The listing builds one solid part. Answer for the finished solid, in the listing's coordinates (mm). Face numbers are marked on the shaded views. A direction names the side the tool comes from. Coordinates: 2 decimals unless noted, no trailing zeros. Order: outer loops, then holes, each group sorted by start corner. A loop starts at its lowest first (then second) coordinate and runs counter-clockwise, first axis right, second up. Notation, with made-up numbers: (58, 19.5) -> (91, 19.5) arc R34 cw to (91, 50.5) -> close; hole circle Ø11 at (-16.75, 63.25). An arc over 180 degrees is marked (long way). Answer in a Markdown table with one row per item.
```python
from build123d import *

# Parameters (mm, degrees)
SKETCH1_W                       = 16
SKETCH1_H                       = 8
BOSS_EXTRUDE1_DEPTH             = 3
SHELL1_T                        = -1
BOSS_EXTRUDE2_DEPTH             = 11
CUT_EXTRUDE1_DEPTH              = 13
SKETCH4_R                       = 1.2
BOSS_EXTRUDE3_DEPTH             = 3
BOSS_EXTRUDE3_DIRECTION_2_REACH = 8.299


with BuildPart() as part:
    # Sketch1 → Boss-Extrude1 (new body)
    with BuildSketch(Plane(origin=(0, 0, 0), x_dir=(1, 0, 0), z_dir=(0, 1, 0))):
        Rectangle(SKETCH1_W, SKETCH1_H)
    extrude(amount=BOSS_EXTRUDE1_DEPTH)

    # Shell1
    shell1_openings = [part.faces().sort_by_distance(p)[0] for p in [
        (0, 0, 0),
    ]]
    offset(amount=SHELL1_T, openings=shell1_openings, kind=Kind.INTERSECTION)

    # Sketch2 → Boss-Extrude2 (add)
    with BuildSketch(Plane(origin=(0, 3, 0), x_dir=(1, 0, 0), z_dir=(0, 1, 0))):
        with BuildLine():
            Line((-4, 4), (4, 4))
            Line((4, 4), (4, 2.5))
            Line((4, 2.5), (2, 2.5))
            ThreePointArc((2, 2.5), (0, 1.5), (-2, 2.5))
            Line((-2, 2.5), (-4, 2.5))
            Line((-4, 2.5), (-4, 4))
        make_face()
    extrude(amount=BOSS_EXTRUDE2_DEPTH)

    # Sketch3 → Cut-Extrude1 (cut, through all)
    with BuildSketch(Plane(origin=(4, 0, 0), x_dir=(0, 0, -1), z_dir=(1, 0, 0))):
        Polygon((1.5, 14), (1.5, 10), (3.25, 14), align=None)
    extrude(amount=-CUT_EXTRUDE1_DEPTH, mode=Mode.SUBTRACT)

    # Sketch4 → Boss-Extrude3 (add)
    with BuildSketch(Plane(origin=(0, 1.055737705, 2.413114754), x_dir=(1, 0, 0), z_dir=(0, 0.400818834, 0.916157335))):
        with Locations((0, 13.193478025)):
            Circle(SKETCH4_R)
    extrude(amount=BOSS_EXTRUDE3_DEPTH)

    # Sketch4 → Boss-Extrude3 direction 2 (add, up to next)
    with BuildSketch(Plane(origin=(0, 1.055737705, 2.413114754), x_dir=(1, 0, 0), z_dir=(0, 0.400818834, 0.916157335)), mode=Mode.PRIVATE) as boss_extrude3_direction_2_sk1:
        with Locations((0, 13.193478025)):
            Circle(SKETCH4_R)
    boss_extrude3_direction_2_tool1 = extrude(boss_extrude3_direction_2_sk1.sketch, amount=-BOSS_EXTRUDE3_DIRECTION_2_REACH, mode=Mode.PRIVATE) - part.part
    add(boss_extrude3_direction_2_tool1.solids().sort_by_distance((0, 13.143039, -2.87508))[0])


solid = part.part
```
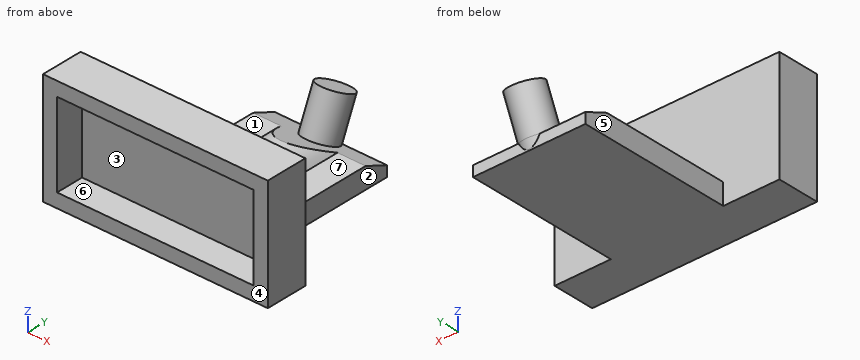
(1) Which of the six approach directions +Z, -Z, +X, -X, +Y, -Y give full straight-line access (tool end or side, diameter ignored) to the marked faces 4, 5, 6 and 7?
Check values:
| item | result |
|---|---|
| face 4 | +Z, -Z, +X, -X, -Y |
| face 5 | +Z, -Z, -X, +Y |
| face 6 | -Y |
| face 7 | +Z, +X, +Y |
(2) A cutting plane is placed at D-D, the plane y = 5.25. Determine the outline of the cut face in (x, z).
Check values:
| item | result |
|---|---|
| outline | (-4, -4) -> (4, -4) -> (4, -2.5) -> (2, -2.5) arc R2.5 ccw to (-2, -2.5) -> (-4, -2.5) -> close |
(3) For a pull along Z with two mould halves and no side action, classify the marked faces 1, 2 and 3 as released by +Z, released by -Z, zero draft, split by the parting line, or undercut.
Check values:
| item | result |
|---|---|
| face 1 | released by +Z |
| face 2 | zero draft |
| face 3 | undercut |
(4) A cutting plane is placed at C-C, the plane z = 2. Determine the outline of the cut face in (x, y), then the cut area to 3 significant figures.
Check values:
| item | result |
|---|---|
| outline | (-8, 0) -> (-7, 0) -> (-7, 2) -> (7, 2) -> (7, 0) -> (8, 0) -> (8, 3) -> (-8, 3) -> close |
| area | 20.0 mm² |
(5) Flat-ended cylindrical pins translate along their axes: pin 1 (4 mm diameter, centred on x = -1.5, z = 0, fed in from -Y); pin 2 (2 mm diameter, centred on x = 4, y = 7.5, fed in from +Z); pin 3 (0.5 mm diameter, centred on y = 11, z = -3.5, fed in from +X). Find the tip coordinate at first contact, or state that the pin passes through.
Check values:
| item | result |
|---|---|
| pin 1 | y = 2 |
| pin 2 | z = -2.5 |
| pin 3 | x = 4 |
(6) Find the intervals of material crossed by line 1 along X through (y, z) = (1, -0.25); line 2 along Y through (x, z) = (-3, 0.75); line 3 along Z through (x, y) = (-0.5, 1.5), in increasing order. Write a range as from..to.
Check values:
| item | result |
|---|---|
| line 1 | -8..-7, 7..8 |
| line 2 | 2..3 |
| line 3 | -4..-3, 3..4 |
(7) A cutting plane is placed at B-B, the plane x = -6. Determine the outline of the cut face in (y, z), then the cut area to 3 significant figures.
Check values:
| item | result |
|---|---|
| outline | (0, -4) -> (3, -4) -> (3, 4) -> (0, 4) -> (0, 3) -> (2, 3) -> (2, -3) -> (0, -3) -> close |
| area | 12.0 mm² |
(8) A cutting plane is placed at A-A, the plane y = 1.25. Determine the outline of the cut face in (x, z), then the cut area to 3 significant figures.
Check values:
| item | result |
|---|---|
| outline | (-8, -4) -> (8, -4) -> (8, 4) -> (-8, 4) -> close; hole (-7, -3) -> (7, -3) -> (7, 3) -> (-7, 3) -> close |
| area | 44.0 mm² |
